```python
from build123d import *

# Parameters (mm, degrees)
SKETCH1_W                    = 38
SKETCH1_H                    = 38
BOSS_EXTRUDE1_DEPTH          = 9.525
F_36_0_1065_DIAMETER_HOLE2_D = 2.7051
SKETCH7_W                    = 8.89
SKETCH7_H                    = 5.08
CUT_EXTRUDE1_DEPTH           = 29.508343077
SKETCH8_W                    = 76.2
SKETCH8_H                    = 9.525
BOSS_EXTRUDE2_DEPTH          = 25.4
F_9_0_196_DIAMETER_HOLE1_D   = 4.9784
FILLET1_R                    = 2.54


with BuildPart() as part:
    # Sketch1 → Boss-Extrude1 (new body)
    with BuildSketch(Plane(origin=(0, 0, 0), x_dir=(0, 1, 0), z_dir=(0, 0, 1))):
        Rectangle(SKETCH1_W, SKETCH1_H)
    extrude(amount=BOSS_EXTRUDE1_DEPTH)

    # #36 (0.1065) Diameter Hole2 (through all)
    with Locations(Plane.XY.offset(9.525)):
        with Locations((-14, -14), (14, -14), (14, 14), (-14, 14)):
            Hole(F_36_0_1065_DIAMETER_HOLE2_D / 2)

    # Sketch7 → Cut-Extrude1 (cut, through all)
    with BuildSketch(Plane(origin=(0, 0, 0), x_dir=(1, 0, 0), z_dir=(0, 0, -1))):
        with Locations((7.05999991, 13.629999978)):
            Rectangle(SKETCH7_W, SKETCH7_H)
    extrude(amount=-CUT_EXTRUDE1_DEPTH, mode=Mode.SUBTRACT)

    # Sketch8 → Boss-Extrude2 (add)
    with BuildSketch(Plane(origin=(0, 19, 0), x_dir=(-1, 0, 0), z_dir=(0, 1, 0))):
        with Locations((0, 4.7625)):
            Rectangle(SKETCH8_W, SKETCH8_H)
    extrude(amount=BOSS_EXTRUDE2_DEPTH)

    # #9 (0.196) Diameter Hole1 (through all)
    with Locations(Plane(origin=(0, 0, 0), x_dir=(1, 0, 0), z_dir=(0, 0, -1))):
        with Locations((-25.4, -31.7), (-12.7, -31.7), (0, -31.7), (12.7, -31.7), (25.4, -31.7)):
            Hole(F_9_0_196_DIAMETER_HOLE1_D / 2)

    # Fillet1
    fillet1_edges = [part.edges().sort_by_distance(p)[0] for p in [
        (-38.1, 19, 4.7625),
        (38.1, 19, 4.7625),
        (-38.1, 44.4, 4.7625),
        (38.1, 44.4, 4.7625),
        (19, 19, 4.7625),
        (19, -19, 4.7625),
        (-19, -19, 4.7625),
        (-19, 19, 4.7625),
    ]]
    fillet(fillet1_edges, radius=FILLET1_R)


solid = part.part
```
Can you work these out from the model? Positions are in its coordinate system, mm. A direction names the side the tool comes from. Round coordinates to 2 decimals unless told otherwise and drop trailing zeros. Loops run counter-clockwise (first coordinate to the right, second up) from the corner with the lowest first, then second, coordinate; pieces in that order, holes last. Notation, with made-up numbers: (-33, -35.75) -> (-12, -35.75) arc R19 ccw to (-12, -15.75) -> close; hole circle Ø4 at (62, 65.25). An arc over 180 degrees is marked (long way). Answer in a Markdown table with one row per item.
Item 1: If I drill on probe 1 along X at (y, z) = (31.7, 7); probe 2 along Y at (x, z) = (6.5, 6.75); probe 3 along Y at (x, z) = (25.4, 4.75), over which ranges is the centre line in solid material (lowest first)?
Answer block:
| item | result |
|---|---|
| probe 1 | -38.1 to -27.89, -22.91 to -15.19, -10.21 to -2.49, 2.49 to 10.21, 15.19 to 22.91, 27.89 to 38.1 |
| probe 2 | -19 to -16.17, -11.09 to 44.4 |
| probe 3 | 19 to 29.21, 34.19 to 44.4 |
Item 2: Suppose I cut it at A-A, the plane x = -25.4. List the corners of the cut face in (y, z) for me (3 decimals).
Answer block:
| item | result |
|---|---|
| outline | (19, 0) -> (29.211, 0) -> (29.211, 9.525) -> (19, 9.525) -> close; (34.189, 0) -> (44.4, 0) -> (44.4, 9.525) -> (34.189, 9.525) -> close |
Item 3: Will these pins go through, and if not, where does the flat tip stop? P1, Ø1, axis at y = 11.5, z = 1, coming from the -X side; P2, Ø4, axis at y = -14.5, z = 3.5, coming from the +X side; P3, Ø3, axis at x = 30.5, z = 6, coming from the -Y side.
Answer block:
| item | result |
|---|---|
| P1 | x = -19 |
| P2 | x = 19 |
| P3 | y = 19 |
Item 4: Suppose I cut it at D-D, the plane y = 31.7. List the corners of the cut face in (x, z) for me (3 decimals).
Answer block:
| item | result |
|---|---|
| outline | (-38.1, 0) -> (-27.889, 0) -> (-27.889, 9.525) -> (-38.1, 9.525) -> close; (-22.911, 0) -> (-15.189, 0) -> (-15.189, 9.525) -> (-22.911, 9.525) -> close; (-10.211, 0) -> (-2.489, 0) -> (-2.489, 9.525) -> (-10.211, 9.525) -> close; (2.489, 0) -> (10.211, 0) -> (10.211, 9.525) -> (2.489, 9.525) -> close; (15.189, 0) -> (22.911, 0) -> (22.911, 9.525) -> (15.189, 9.525) -> close; (27.889, 0) -> (38.1, 0) -> (38.1, 9.525) -> (27.889, 9.525) -> close |
Item 5: Suppose I cut it at B-B, the plane y = -14. List the corners of the cut face in (x, z) for me (3 decimals).
Answer block:
| item | result |
|---|---|
| outline | (-19, 0) -> (-15.353, 0) -> (-15.353, 9.525) -> (-19, 9.525) -> close; (-12.647, 0) -> (2.615, 0) -> (2.615, 9.525) -> (-12.647, 9.525) -> close; (11.505, 0) -> (12.647, 0) -> (12.647, 9.525) -> (11.505, 9.525) -> close; (15.353, 0) -> (19, 0) -> (19, 9.525) -> (15.353, 9.525) -> close |
Item 6: We'd pull the mould along X, two halves only. Please class faces 1 (the cylindrical face through (19.764, 18.276, 4.829)), 2 (the cylindrical face through (-37.376, 19.764, 4.829)), 3 (the cylindrical face through (-12.38, 29.23, 4.83)), 4 (the flat face through (7, -16.17, 5)): released by +X, released by -X, zero draft, split by the parting line, or undercut.
Answer block:
| item | result |
|---|---|
| face 1 | released by +X |
| face 2 | released by -X |
| face 3 | undercut |
| face 4 | undercut |
Item 7: Suppose I cut it at C-C, the plane z = 8.25. Give the number of separate pieces and of enclosed holes in the cut face, plus the area to 3 significant figures.
Answer block:
| item | result |
|---|---|
| separate pieces | 1 |
| enclosed holes | 10 |
| area | 3,210 mm² |
Item 8: On a 3-axis mill with a long thin cutter (end or side, diameter ignored), from which of +Z, -Z, +X, -X, +Y, -Y can I reach the whole of each face in a straight line? I mean faces 5 (the flat face through (11.505, -14, 5)), 6 (the flat face through (29, 19, 5)), 7 (the flat face through (-38.1, 32, 5)). Say none if no direction works.
Answer block:
| item | result |
|---|---|
| face 5 | +Z, -Z |
| face 6 | +Z, -Z, +X, -Y |
| face 7 | +Z, -Z, -X, +Y, -Y |
